Geometry: final body of the model. Coordinates: model frame, mm. Face numbers are marked on the shaded views. Round coordinates to 2 decimals unless told otherwise and drop trailing zeros. Order: outer loops, then holes, each group sorted by start corner. A loop starts at its lowest first (then second) coordinate and runs counter-clockwise, first axis right, second up. Notation, with made-up numbers: M 6.5,6.5 L 48.5,6.5 A20 ccw 48.5,33.5 Z; hole C 81.25,-15 d5. An arc over 180 degrees is marked long. Return JSON: item names as keys, results as strings. Group by question number.
Q1. Cut plane C-C on y = 3.75. Output: boundary loops of the cut face in (x, z) (3 decimals), and give its area (3 significant figures).
Q2. Cut plane A-A on x = 0. Output: boundary loops of the cut face in (y, z) (3 decimals).
Q3. Cut plane D-D on x = 148. Output: boundary loops of the cut face in (y, z), and give its area (3 significant figures).
Q4. Mould query, pull axis Y, two halves, no side actions, for the marked faces 1 and 2. Classes: released by +Y, released by -Y, zero draft, split by the parting line, or undercut.
Q5. Contact query for flat-ended pins moving along their axis: pin 1 (3 mm diameter, centred on y = 2, z = 34, fed in from -X); pin 2 (1.9 mm diameter, centred on x = 144.5, y = 4.5, fed in from +Z); pin 3 (1.5 mm diameter, centred on x = -2.5, y = 4.5, fed in from -Z). Output: stop coordinate, or through.
Q6. Cut plane B-B on z = 0. Output: boundary loops of the cut face in (x, y) (3 decimals), and give its area (3 significant figures).
Q7. Ray query, probe 1 along X at (y, z) = (4, 0) (3 decimals); probe 2 along Z at (x, y) = (-174, 5.75); probe 3 along X at (y, z) = (4.25, 22.5). Return the intervals inside material, ascending.
```python
from build123d import *

# Parameters (mm, degrees)
SKETCH1_R           = 53.975
BOSS_EXTRUDE1_DEPTH = 6.35
FILLET1_R           = 3.175


with BuildPart() as part:
    # Sketch1 → Boss-Extrude1 (new body)
    with BuildSketch(Plane(origin=(0, 0, 0), x_dir=(1, 0, 0), z_dir=(0, 1, 0))):
        with BuildLine():
            Line((65.454301807, 12.7), (190.5, 12.7))
            Line((190.5, 12.7), (190.5, -12.7))
            Line((190.5, -12.7), (65.454301807, -12.7))
            ThreePointArc((65.454301807, -12.7), (0, -66.675), (-65.454301807, -12.7))
            Line((-65.454301807, -12.7), (-190.5, -12.7))
            Line((-190.5, -12.7), (-190.5, 12.7))
            Line((-190.5, 12.7), (-65.454301807, 12.7))
            ThreePointArc((-65.454301807, 12.7), (0, 66.675), (65.454301807, 12.7))
        make_face()
        with Locations(Location((0, 0, 0), (0, 0, 270))):
            Circle(SKETCH1_R, mode=Mode.SUBTRACT)
    extrude(amount=BOSS_EXTRUDE1_DEPTH)

    # Fillet1
    fillet1_edges = [part.edges().sort_by_distance(p)[0] for p in [
        (65.454301807, 3.175, 12.7),
        (-65.454301807, 3.175, 12.7),
        (-65.454301807, 3.175, -12.7),
        (65.454301807, 3.175, -12.7),
    ]]
    fillet(fillet1_edges, radius=FILLET1_R)


solid = part.part
```
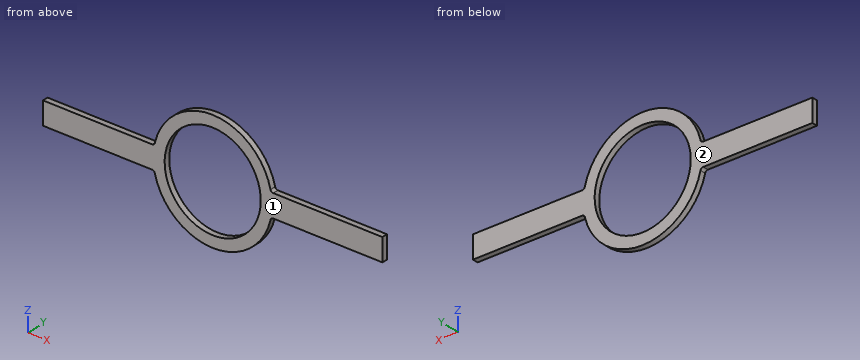
Result sheet:
{
 "1": {"outline": "M -190.5,-12.7 L -68.022,-12.7 A3.175 cw -64.93,-15.153 A66.675 ccw 64.93,-15.153 A3.175 cw 68.022,-12.7 L 190.5,-12.7 L 190.5,12.7 L 68.022,12.7 A3.175 cw 64.93,15.153 A66.675 ccw -64.93,15.153 A3.175 cw -68.022,12.7 L -190.5,12.7 Z; hole C 0,0 d107.95", "area": "11,100 mm²"},
 "2": {"outline": "M 0,-66.675 L 6.35,-66.675 L 6.35,-53.975 L 0,-53.975 Z; M 0,53.975 L 6.35,53.975 L 6.35,66.675 L 0,66.675 Z"},
 "3": {"outline": "M 0,-12.7 L 6.35,-12.7 L 6.35,12.7 L 0,12.7 Z", "area": "161 mm²"},
 "4": {"face 1": "released by -Y", "face 2": "released by +Y"},
 "5": {"pin 1": "stops at x = -58.22", "pin 2": "stops at z = 12.7", "pin 3": "stops at z = -66.65"},
 "6": {"outline": "M -190.5,0 L -53.975,0 L -53.975,6.35 L -190.5,6.35 Z; M 53.975,0 L 190.5,0 L 190.5,6.35 L 53.975,6.35 Z", "area": "1,730 mm²"},
 "7": {"probe 1": "x = -190.5 to -53.975, 53.975 to 190.5", "probe 2": "z = -12.7 to 12.7", "probe 3": "x = -62.76 to -49.06, 49.06 to 62.76"}
}
